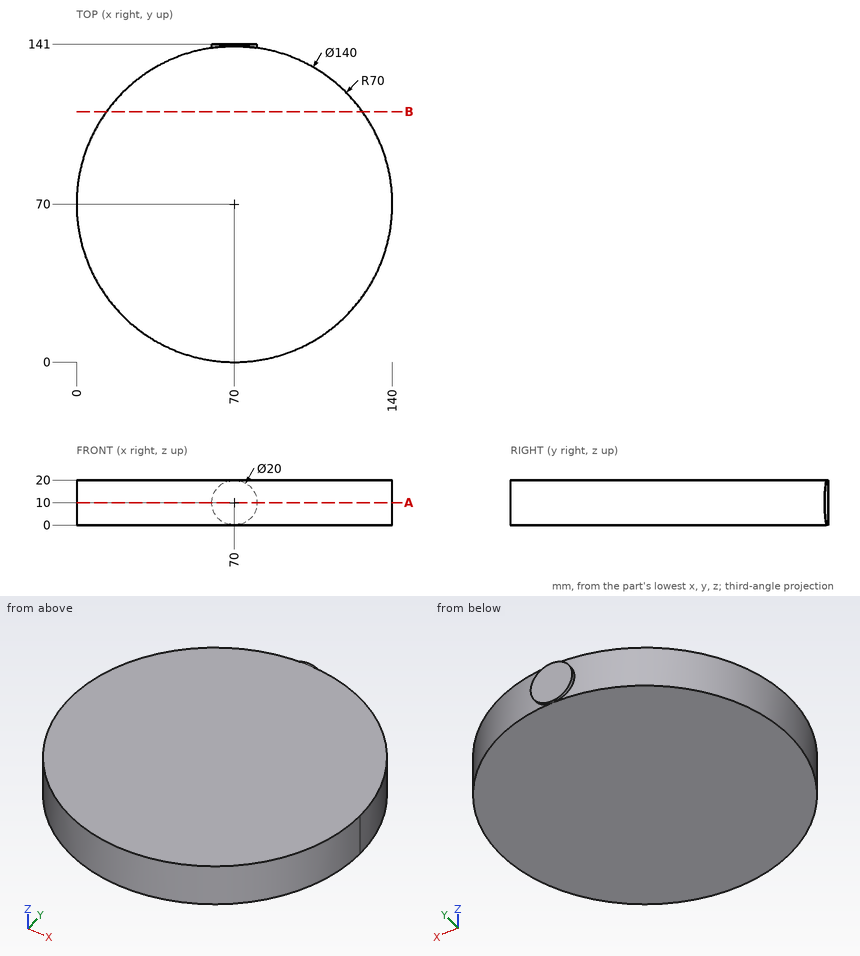
Here's the drawing with two shaded views (mm, measured from the low corner). I have some questions. Round coordinates to 2 decimals unless told otherwise and drop trailing zeros. Loops run counter-clockwise (first coordinate to the right, second up) from the corner with the lowest first, then second, coordinate; pieces in that order, holes last. Notation, with made-up numbers: (67, -35.75) - (100, -35.75) arc R18 ccw to (100, -28.75) - close; hole circle Ø1 at (-18.75, -24.75). An arc over 180 degrees is marked (long way). Write item = value, one per line.
1) I need wall thicknesses on line 1 along X through (y, z) = (104.5, 7.5); line 2 along X through (y, z) = (57, 3.5); line 3 along Y through (x, z) = (45, 5). Which ranges of each line are inside material? Lowest first, please. Write a range as from..to.
Computed:
line_1 = 9.09..130.91
line_2 = 1.22..138.78
line_3 = 4.62..135.38
2) Imagine slicing it at A-A (z = 10). Please give me the cut outline in (x, y), and give its area (3 significant figures).
Computed:
outline = (60, 139.28) arc R70 ccw (long way) to (80, 139.28) - (80, 141) - (60, 141) - close
area = 15,400 mm2
3) Imagine slicing it at B-B (y = 111). Please give me the cut outline in (x, z).
Computed:
outline = (13.26, 0) - (126.74, 0) - (126.74, 20) - (13.26, 20) - close
4) I'm going to push flat-ended pins straight in: P1, Ø2, axis at y = 120, z = 14, coming from the -X side; P2, Ø4, axis at x = 15, z = 5, coming from the -Y side; P3, Ø12, axis at y = 115, z = 13.5, coming from the +X side. Where does each tip first touch, or does it pass through?
Computed:
P1 = 20.01
P2 = 24.27
P3 = 128.13
